Geometry check sheet. Reference: the model listing, model coordinates, mm. Face numbers are marked on the shaded views. A direction names the side the tool comes from. Round coordinates to 2 decimals unless told otherwise and drop trailing zeros. Loops run counter-clockwise (first coordinate to the right, second up) from the corner with the lowest first, then second, coordinate; pieces in that order, holes last. Notation, with made-up numbers: (10.5, 28) - (50.5, 28) arc R24 cw to (50.5, 49) - close; hole circle Ø4 at (-39, 80.25). An arc over 180 degrees is marked (long way). Write item = value, one per line.
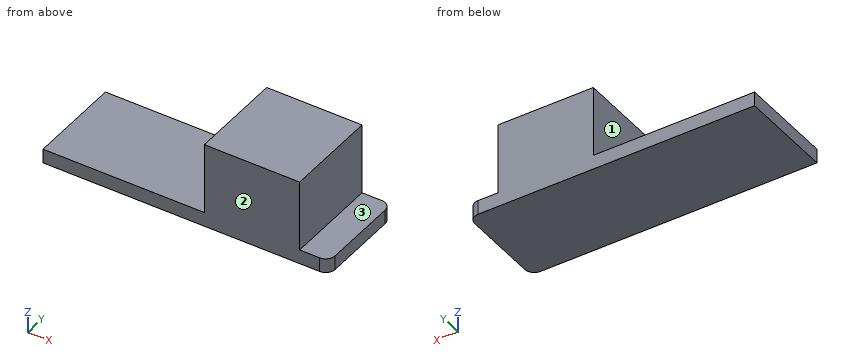
```python
from build123d import *

# Parameters (mm, degrees)
F0_W     = 50.8
F0_H     = 37.8133962381
F0_H_2   = 0.2866037619
F1_DEPTH = 50.8
F2_R     = 5.08


with BuildPart() as f1:
    # F0 (on Front) → F1 (new body)
    with BuildSketch(Plane.XZ):
        with Locations((0, 0.143301881)):
            Rectangle(F0_W, F0_H)
        with Locations((0, -18.906698119)):
            Rectangle(F0_W, F0_H_2)
        Polygon((-25.4, -19.05), (-25.4, -18.7633962381), (-111.351557076, -18.7633962381), (-111.351557076, -26.3833962381), (41.048442924, -26.3833962381), (41.048442924, -18.7633962381), (25.4, -18.7633962381), (25.4, -19.05), align=None)
    extrude(amount=F1_DEPTH)

    # F2
    f2_edges = [f1.edges().sort_by_distance(p)[0] for p in [
        (41.048443, 0, -22.573396),
        (41.048443, -50.8, -22.573396),
    ]]
    fillet(f2_edges, radius=F2_R)


solid = f1.part
```
(1) Gauge pin test, flat ends, axial feed: pin 1 (12 mm diameter, centred on y = -18, z = -5, fed in from +X); pin 2 (2 mm diameter, centred on y = -39, z = 2, fed in from -X); pin 3 (8 mm diameter, centred on x = 31, y = -21, fed in from +Z). Record the tip position at first contact, or that the pin passes through.
Answers follow:
pin_1 = 25.4
pin_2 = -25.4
pin_3 = -18.76
(2) Scan lines: L1, parallel to X at y = -5, z = 0; L2, parallel to Z at x = -45, y = -9.5. Record each from-to range of solid material in increasing order. Write a range as [from, to].
Answers follow:
L1 = [-25.4, 25.4]
L2 = [-26.38, -18.76]
(3) Set-up check for the marked faces 1, 2 and 3: record each of +Z, -Z, +X, -X, +Y, -Y from which the full face is reachable in a straight line by a thin tool's end or side.
Answers follow:
face_1 = +Z, -X, +Y, -Y
face_2 = +Z, -Z, +X, -X, -Y
face_3 = +Z, +X, +Y, -Y
(4) Section check C-C (z = -15.5). Enter the section's corners in (x, y).
Answers follow:
outline = (-25.4, -50.8) - (25.4, -50.8) - (25.4, 0) - (-25.4, 0) - close
(5) Section check A-A (y = -27). Enter the section's corners in (x, z).
Answers follow:
outline = (-111.35, -26.38) - (41.05, -26.38) - (41.05, -18.76) - (25.4, -18.76) - (25.4, 19.05) - (-25.4, 19.05) - (-25.4, -18.76) - (-111.35, -18.76) - close
(6) Section check B-B (x = -35.5). Enter the section's corners in (y, z), then the cut area to 3 significant figures.
Answers follow:
outline = (-50.8, -26.38) - (0, -26.38) - (0, -18.76) - (-50.8, -18.76) - close
area = 387 mm²
